Verification items for the finished model (mm, model axes). Give positions to 0.01 mm unless a question says otherwise; leave off trailing zeros. Order: outer loops, then holes, each group sorted by start corner. A loop starts at its lowest first (then second) coordinate and runs counter-clockwise, first axis right, second up. Notation, with made-up numbers: M 85,33.5 L 106,33.5 A22 ccw 106,49.5 Z; hole C -27,41.5 d1. An arc over 180 degrees is marked long. Answer as a JSON object with one key per item and string values.
```python
from build123d import *

# Parameters (mm, degrees)
SKETCH1_W           = 73
SKETCH1_H           = 29
BOSS_EXTRUDE1_DEPTH = 5
SKETCH2_R           = 1
CUT_EXTRUDE1_DEPTH  = 35


with BuildPart() as part:
    # Sketch1 → Boss-Extrude1 (new body)
    with BuildSketch(Plane.XY):
        with Locations((36.5, 14.5)):
            Rectangle(SKETCH1_W, SKETCH1_H)
        Polygon((-10, 29), (0, 29), (5, 29), (5, 33), (-10, 33), align=None)
        Polygon((5, 0), (0, 0), (-10, 0), (-10, -4), (5, -4), align=None)
    extrude(amount=BOSS_EXTRUDE1_DEPTH)

    # Sketch2 → Cut-Extrude1 (cut)
    with BuildSketch(Plane(origin=(0, 33, 0), x_dir=(1, 0, 0), z_dir=(0, 1, 0))):
        with Locations(Location((-7, -2.46940408, 0), (0, 0, 270))):
            Circle(SKETCH2_R)
    extrude(amount=-CUT_EXTRUDE1_DEPTH, mode=Mode.SUBTRACT)


solid = part.part
```
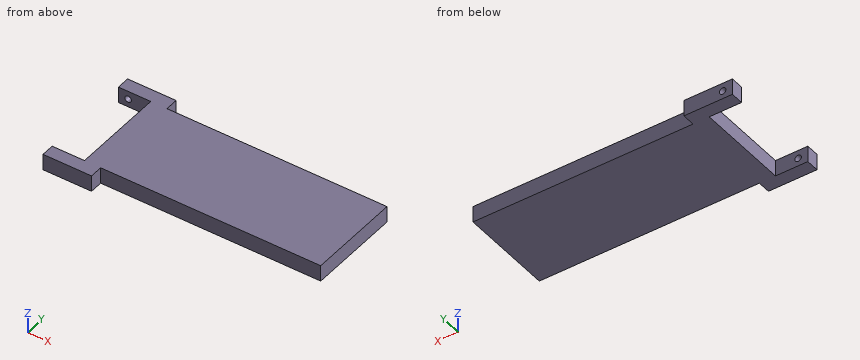
Q1. Section check C-C on x = 53.5. Record the cut outline in (y, z), then the cut area to 3 significant figures.
Resolved:
{"outline": "M 0,0 L 29,0 L 29,5 L 0,5 Z", "area": "145 mm²"}
Q2. Gauge pin test, flat ends, axial feed: pin 1 Ø3 at (y, z) = (32, 3) entering from +X; pin 2 Ø1 at (x, z) = (63, 0.5) entering from +Y; pin 3 Ø1 at (x, z) = (57.5, 3) entering from -Y. Record the tip position at first contact, or that the pin passes through.
Resolved:
{"pin 1": "stops at x = 5", "pin 2": "stops at y = 29", "pin 3": "stops at y = 0"}
Q3. Section check B-B on y = 17. Record the cut outline in (x, z).
Resolved:
{"outline": "M 0,0 L 73,0 L 73,5 L 0,5 Z"}
Q4. Section check A-A on x = -7. Record the cut outline in (y, z), then the cut area to 3 significant figures.
Resolved:
{"outline": "M -4,0 L 0,0 L 0,1.47 L -2,1.47 L -2,3.47 L 0,3.47 L 0,5 L -4,5 Z; M 29,0 L 33,0 L 33,1.47 L 29,1.47 Z; M 29,3.47 L 33,3.47 L 33,5 L 29,5 Z", "area": "28.0 mm²"}
Q5. Material ranges on L1, parallel to Y at x = 34, z = 4.1; L2, parallel to X at y = 14, z = 3.6; L3, parallel to Y at x = -6.5, z = 3.15, recorded low to high.
Resolved:
{"L1": "y = 0 to 29", "L2": "x = 0 to 73", "L3": "y = -4 to -2"}
